from build123d import *

# Parameters (mm, degrees)
SKETCH1_W                                         = 88
SKETCH1_H                                         = 70
BOSS_EXTRUDE2_DEPTH                               = 1.5
SKETCH7_W                                         = 86
SKETCH7_H                                         = 68
BOSS_EXTRUDE3_DEPTH                               = 1
CSK_FOR_M2_5_FLAT_HEAD_MACHINE_SCREW1_D           = 2.9
CSK_FOR_M2_5_FLAT_HEAD_MACHINE_SCREW1_DEPTH       = 2.128752102
CSK_FOR_M2_5_FLAT_HEAD_MACHINE_SCREW1_CSINK_D     = 5.5
CSK_FOR_M2_5_FLAT_HEAD_MACHINE_SCREW1_CSINK_ANGLE = 90
CSK_FOR_M2_5_FLAT_HEAD_MACHINE_SCREW1_TIP         = 0.871247898


with BuildPart() as part:
    # Sketch1 → Boss-Extrude2 (new body)
    with BuildSketch(Plane(origin=(0, 0, 0), x_dir=(1, 0, 0), z_dir=(0, 1, 0))):
        Rectangle(SKETCH1_W, SKETCH1_H)
    extrude(amount=BOSS_EXTRUDE2_DEPTH)

    # Sketch7 → Boss-Extrude3 (add)
    with BuildSketch(Plane(origin=(0, 1.5, 0), x_dir=(1, 0, 0), z_dir=(0, 1, 0))):
        Rectangle(SKETCH7_W, SKETCH7_H)
    extrude(amount=BOSS_EXTRUDE3_DEPTH)

    # CSK for M2.5 Flat Head Machine Screw1
    with Locations(Plane(origin=(0, 0, 0), x_dir=(-1, 0, 0), z_dir=(0, -1, 0))):
        with Locations((-40, -32), (-41, 31), (31.5, 31), (40.268, -32)):
            CounterSinkHole(CSK_FOR_M2_5_FLAT_HEAD_MACHINE_SCREW1_D / 2, CSK_FOR_M2_5_FLAT_HEAD_MACHINE_SCREW1_CSINK_D / 2, depth=CSK_FOR_M2_5_FLAT_HEAD_MACHINE_SCREW1_DEPTH, counter_sink_angle=CSK_FOR_M2_5_FLAT_HEAD_MACHINE_SCREW1_CSINK_ANGLE)
            with Locations((0, 0, -(CSK_FOR_M2_5_FLAT_HEAD_MACHINE_SCREW1_DEPTH + CSK_FOR_M2_5_FLAT_HEAD_MACHINE_SCREW1_TIP / 2))):  # 118° drill point
                Cone(0, CSK_FOR_M2_5_FLAT_HEAD_MACHINE_SCREW1_D / 2, CSK_FOR_M2_5_FLAT_HEAD_MACHINE_SCREW1_TIP, mode=Mode.SUBTRACT)


solid = part.part
Geometry check sheet. Reference: the model listing, model coordinates, mm. A direction names the side the tool comes from. Give positions to 0.01 mm unless a question says otherwise; leave off trailing zeros. Write each loop counter-clockwise with the first axis right and the second up, starting at its lowest first coordinate (ties: lowest second). Pieces come first, ordered by that corner, then holes. Notation, with made-up numbers: M 43,60 L 97,60 A4 ccw 97,64 Z; hole C 27,-23.5 d2. An arc over 180 degrees is marked long. Answer as CSV lines item,"result". Start each with the question number.
Q1. Release check for a two-part mould opening along Z. For faces 3 (the face through (-30.831, 1.72, -29.714)), 4 (the face through (-1, 0, 0)) record: pulls with the +Z half, pulls with the -Z half, needs draft (parallel to the pull), parting line crosses it, or undercut.
Q2. Go/stop test with a flat-tipped pin: pin 1 (3.5 mm diameter, centred on x = -31.5, z = -31, fed in from -Y). Record where the tip stops, or that it passes through.
Q3. Tool access check on faces 1 (the face through (-1, 2.5, 0)), 2 (the face through (39.85, 1.72, -30.12)). Record the directions out of +Z, -Z, +X, -X, +Y, -Y that give a thin tool (end or side, any length) a straight path to the whole face; none if there is none.
Q4. Material ranges on L1, parallel to X at y = 1.95, z = -31; L2, parallel to X at y = 1.6, z = 32; L3, parallel to Z at x = 40, y = 1.65, recorded low to high.
Q5. Section check A-A, the plane z = 32. Record the cut outline in (x, y), then the cut area to 3 significant figures.
Geometry says:
1,face 3,"undercut"
1,face 4,"needs draft"
2,pin 1,"y = 1"
3,face 1,"+Z, -Z, +X, -X, +Y"
3,face 2,"-Y"
4,L1,"-43 to -32.95, -30.05 to 39.55, 42.45 to 43"
4,L2,"-43 to -41.72, -38.82 to 38.55, 41.45 to 43"
4,L3,"-34 to -32.05, -29.95 to 30.55, 33.45 to 34"
5,outline,"M -44,0 L -43.02,0 L -41.72,1.3 L -41.72,2.13 L -41.1,2.5 L -43,2.5 L -43,1.5 L -44,1.5 Z; M -39.44,2.5 L -38.82,2.13 L -38.82,1.3 L -37.52,0 L 37.25,0 L 38.55,1.3 L 38.55,2.13 L 39.17,2.5 Z; M 40.83,2.5 L 41.45,2.13 L 41.45,1.3 L 42.75,0 L 44,0 L 44,1.5 L 43,1.5 L 43,2.5 Z"
5,area,"201 mm^2"
